Part model, mm, in its own coordinate system. A direction names the side the tool comes from. Give positions to 0.01 mm unless a question says otherwise; leave off trailing zeros. Loops run counter-clockwise (first coordinate to the right, second up) from the corner with the lowest first, then second, coordinate; pieces in that order, holes last. Notation, with made-up numbers: M 7,-24.75 L 23,-24.75 A30 cw 23,7.25 Z; hole C 4.25,9.25 d7. An arc over 180 degrees is marked long. Put each result on its own line as item: value. Start each with the question number.
```python
from build123d import *

# Parameters (mm, degrees)
F0_R     = 7
F1_DEPTH = 43


with BuildPart() as f1:
    # F0 (on Front) → F1 (new body)
    with BuildSketch(Plane.XZ):
        with BuildLine():
            ThreePointArc((-20.091246, -9.108256), (-17.950626, -18.121598), (-13.076884, -26))
            Line((-13.076884, -26), (-7.864951, -26))
            Line((-7.864951, -26), (21.135049, 7))
            Line((21.135049, 7), (21.135049, 26))
            Line((21.135049, 26), (16.135049, 31))
            Line((16.135049, 31), (-7.864951, 31))
            ThreePointArc((-7.864951, 31), (-16.289978, 23.276069), (-27.621866, 21.783252))
            Line((-27.621866, 21.783252), (-45.864951, 25))
            Line((-45.864951, 25), (-52.864951, 25))
            Line((-52.864951, 25), (-59.864951, 18))
            Line((-59.864951, 18), (-59.864951, 0))
            Line((-59.864951, 0), (-52.864951, -7))
            Line((-52.864951, -7), (-24.170194, -7))
            ThreePointArc((-24.170194, -7), (-21.874407, -7.558226), (-20.091246, -9.108256))
        make_face()
        with Locations((-45.864951, 7)):
            Circle(F0_R, mode=Mode.SUBTRACT)
    extrude(amount=F1_DEPTH)


solid = f1.part
```
1) Mould opens along X. For faces 1 (the flat face through (-11, -21, -26)), 2 (the flat face through (-56.316, -21.199, 21.549)), 3 (the flat face through (-36.62, -21.2, 23.37)) say: +X half, -X half, draft (parallel to the pull), parting line (faces both ways), or undercut.
2) Pin check, flat tips, straight feed: pin 1 Ø8 at (x, y) = (1, -37.5) entering from -Z; pin 2 Ø1 at (x, y) = (-25, -5.5) entering from -Z; pin 3 Ø5.5 at (x, y) = (-47.5, -32) entering from +Z. Stop position of each tip, or through.
3) Band-saw the part on A-A on y = -32.5. Give the cut face in (x, z).
4) Which spindle directions (+Z, -Z, +X, -X, +Y, -Y) get a long thin tool onto all of the face, cutting with end or side? Do faces 4 (the flat face through (-20, -43, 9)), 5 (the flat face through (-39, -21, -7)), 6 (the flat face through (-49, -21, 25)). Say none if no direction does.
5) Band-saw the part on D-D on x = 11. Give the cut face in (y, z).
6) Band-saw the part on C-C on z = 23.5. Give the cut face in (x, y), then the cut area to 3 significant figures.
7) Wall check: L1, parallel to Z at x = -46, y = -31; L2, parallel to Z at x = -27.5, y = -30; L3, parallel to X at y = -32.5, z = -16. Give the ranges that are in metal, low to high.
8) Band-saw the part on B-B on z = 2. Give the cut face in (x, y).
Evaluation:
1. face 1: draft
1. face 2: -X half
1. face 3: undercut
2. pin 1: z = -20.46
2. pin 2: z = -7
2. pin 3: z = 25
3. outline: M -59.86,0 L -52.86,-7 L -24.17,-7 A5 cw -20.09,-9.11 A29 ccw -13.08,-26 L -7.86,-26 L 21.14,7 L 21.14,26 L 16.14,31 L -7.86,31 A19 cw -27.62,21.78 L -45.86,25 L -52.86,25 L -59.86,18 Z; hole C -45.86,7 d14
4. face 4: +Z, -Z, +X, -X, -Y
4. face 5: -Z, -X, +Y, -Y
4. face 6: +Z, -X, +Y, -Y
5. outline: M -43,-4.53 L 0,-4.53 L 0,31 L -43,31 Z
6. outline: M -54.36,-43 L -37.36,-43 L -37.36,0 L -54.36,0 Z; M -15.83,-43 L 21.14,-43 L 21.14,0 L -15.83,0 Z
6. area: 2,320 mm2
7. L1: -7 to 0, 14 to 25
7. L2: -7 to 21.76
7. L3: -18.74 to 0.92
8. outline: M -59.86,-43 L -50.76,-43 L -50.76,0 L -59.86,0 Z; M -40.97,-43 L 16.74,-43 L 16.74,0 L -40.97,0 Z
